Read the model definition and answer for the solid it produces. Units are mm, in the model's axes. Face numbers are marked on the shaded views. A direction names the side the tool comes from. Coordinates: 2 decimals unless noted, no trailing zeros. Loops run counter-clockwise (first coordinate to the right, second up) from the corner with the lowest first, then second, coordinate; pieces in that order, holes last. Notation, with made-up numbers: (56.5, 64) -> (110.5, 64) arc R6 ccw to (110.5, 74) -> close; hole circle Ø8 at (-5.5, -17.75). An arc over 180 degrees is marked (long way). Answer as a JSON object with one key per item and string values. Group by question number.
1) Which of the six approach directions +Z, -Z, +X, -X, +Y, -Y give full straight-line access (tool end or side, diameter ignored) to the marked faces 1, 2 and 3?
2) Section C-C, the plane z = 2.5 is taken. Give the vertices of the cut face in (x, y), plus the area to 3 significant figures.
3) Consider probe 1 along Y at (x, z) = (0, 2.65); probe 2 along Y at (x, z) = (0, 0.4); probe 3 along Z at (x, y) = (6.25, 4.25). Determine where each line is inside the solid, lowest interval first. Write a range as [from, to].
4) Section A-A, the plane x = 1.5 is taken. Count the separate pieces of the cut face and the enclosed holes in it, plus the area to 3 significant figures.
5) Determine the mould class of the marked faces 4, 5 and 6 for opening direction X: released by +X, released by -X, zero draft, split by the parting line, or undercut.
6) Section B-B, the plane y = 8.5 is taken. Give the vertices of the cut face in (x, z).
7) Flat-ended cylindrical pins translate along their axes: P1, Ø2, axis at x = -3, z = 7, coming from the +Y side; P2, Ø2, axis at y = 3.5, z = 6.5, coming from the +X side; P3, Ø3, axis at x = -7.15, y = 0, coming from the +Z side; P4, Ø2, axis at x = 0, y = -7.15, coming from the -Z side. Find the tip coordinate at first contact, or state that the pin passes through.
8) Section D-D, the plane y = -7.5 is taken. Give the vertices of the cut face in (x, z).
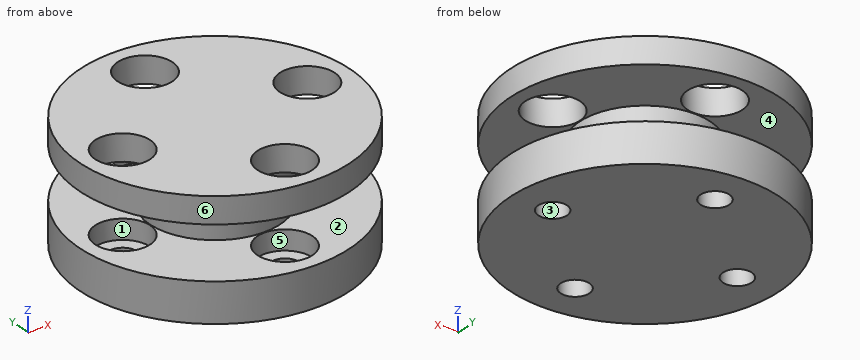
Autodesk Fusion 360 part; units mm, degrees
sketch "Sketch1" plane through (0, 0, 0) normal (0, 0, 1) x (1, 0, 0)
  circle A0 centre (0, 0) radius 10.3
  dimension "d1" = 20.6
extrude "Extrude1" add sketch "Sketch1" along normal blind 3
sketch "Sketch2" plane through (0, 0, 3) normal (0, 0, 1) x (-1, 0, 0)
  circle A0 centre (0, 0) radius 10.3
  circle A1 centre (0, 0) radius 5
  dimension "d4" = 10
extrude "Extrude2" add sketch "Sketch2" along normal blind 4 contours A1
sketch "Sketch3" plane through (0, 0, 7) normal (0, 0, 1) x (-1, 0, 0)
  circle A0 centre (0, 0) radius 5
  circle A1 centre (0, 0) radius 10.3
  dimension "d7" = 20.6
extrude "Extrude3" add sketch "Sketch3" along normal blind 2 contours A0 | A1
sketch "Sketch4" plane through (0, 0, 9) normal (0, 0, 1) x (-1, 0, 0)
  circle A0 centre (0, 0) radius 10.3
  circle A1 centre (-7.15, 0) radius 1.1
  line L0 (0, 0) -> (-7.15, 0)
  dimension "d10" = 2.2
  dimension "d23" = 7.15
extrude "Extrude4" cut sketch "Sketch4" against normal blind 9 contours A1
pattern_circular "C-Pattern1" count 4 over 360 about axis through (0, 0, 7) along (0, 0, 1) of "Extrude4"
sketch "Sketch5" plane through (0, 0, 9) normal (0, 0, 1) x (-1, 0, 0)
  circle A0 centre (0, 7.15) radius 1.1
  circle A1 centre (7.15, 0) radius 1.1
  circle A2 centre (0, -7.15) radius 1.1
  circle A3 centre (-7.15, 0) radius 1.1
  circle A4 centre (0, 0) radius 10.3
  circle A5 centre (0, 7.15) radius 2.1
  dimension "d19" = 4.2
extrude "Extrude5" cut sketch "Sketch5" against normal blind 7.5 contours A5
pattern_circular "C-Pattern2" count 4 over 360 about axis through (0, 0, 3) along (0, 0, 1) of "Extrude5"
hole "Hole1" at (5, 0, 4.7624) direction (-1, 0, 0) diameter 2 depth 10 tip angle 180
Determined:
{
 "1": {"face 1": "+Z", "face 2": "none", "face 3": "+Z, -Z"},
 "2": {"outline": "circle Ø20.6 at (0, 0); hole circle Ø4.2 at (-7.15, 0); hole circle Ø4.2 at (0, -7.15); hole circle Ø4.2 at (0, 7.15); hole circle Ø4.2 at (7.15, 0)", "area": "278 mm²"},
 "3": {"probe 1": "[-10.3, -9.25], [-5.05, 5.05], [9.25, 10.3]", "probe 2": "[-10.3, -8.25], [-6.05, 6.05], [8.25, 10.3]", "probe 3": "[0, 3], [7, 9]"},
 "4": {"separate pieces": "3", "enclosed holes": "1", "area": "116 mm²"},
 "5": {"face 4": "zero draft", "face 5": "undercut", "face 6": "split by the parting line"},
 "6": {"outline": "(-5.82, 0) -> (5.82, 0) -> (5.82, 3) -> (1.61, 3) -> (1.61, 1.5) -> (-1.61, 1.5) -> (-1.61, 3) -> (-5.82, 3) -> close; (-5.82, 7) -> (-1.61, 7) -> (-1.61, 9) -> (-5.82, 9) -> close; (1.61, 7) -> (5.82, 7) -> (5.82, 9) -> (1.61, 9) -> close"},
 "7": {"P1": "y = 10.1", "P2": "x = 9.96", "P3": "z = 1.5", "P4": "through"},
 "8": {"outline": "(-7.06, 0) -> (-1.04, 0) -> (-1.04, 1.5) -> (-2.07, 1.5) -> (-2.07, 3) -> (-7.06, 3) -> close; (-7.06, 7) -> (-2.07, 7) -> (-2.07, 9) -> (-7.06, 9) -> close; (1.04, 0) -> (7.06, 0) -> (7.06, 3) -> (2.07, 3) -> (2.07, 1.5) -> (1.04, 1.5) -> close; (2.07, 7) -> (7.06, 7) -> (7.06, 9) -> (2.07, 9) -> close"}
}
